Study the drawing (mm; zero at the part's minimum x, y, z) and answer. A direction names the side the tool comes from. Give positions to 0.01 mm unless a question says otherwise; leave off trailing zeros. Order: outer loops, then holes, each group sorted by start corner. A loop starts at its lowest first (then second) coordinate and runs counter-clockwise, first axis right, second up. Notation, with made-up numbers: (-4.75, 29) - (45.25, 29) arc R23 cw to (45.25, 58) - close; hole circle Ø5 at (-19.75, -9). An arc over 180 degrees is marked (long way). Write each question's results on one line, items separated by ' | '. Start each with the question number.
1. Flat-ended cylindrical pins translate along their axes: pin 1 (6.5 mm diameter, centred on x = 10, y = 24, fed in from +Z); pin 2 (12 mm diameter, centred on y = 21, z = 6, fed in from +X); pin 3 (2 mm diameter, centred on y = 6.5, z = 11.5, fed in from -X); pin 4 (6 mm diameter, centred on x = 64, y = 24, fed in from -Z). Find the tip coordinate at first contact, or state that the pin passes through.
2. Section A-A (y = 24) is taken. Give the vertices of the cut face in (x, z), and give its area (3 significant figures).
3. Section D-D (y = 6) is taken. Give the vertices of the cut face in (x, z).
4. Section B-B (z = 20) is taken. Give the vertices of the cut face in (x, y).
5. Section C-C (x = 49) is taken. Give the vertices of the cut face in (y, z), and give its area (3 significant figures).
6. Determine the mould class of the marked faces 4, 5, 6 and 7 for opening direction X: released by +X, released by -X, zero draft, split by the parting line, or undercut.
7. Find the intervals of material crossed by L1, parallel to Y at x = 49, z = 0.9; L2, parallel to X at y = 16.75, z = 16; L3, parallel to Z at x = 28, y = 24.5, in increasing order.
8. Which of the six approach directions +Z, -Z, +X, -X, +Y, -Y give full straight-line access (tool end or side, diameter ignored) to the marked faces 1, 2 and 3?
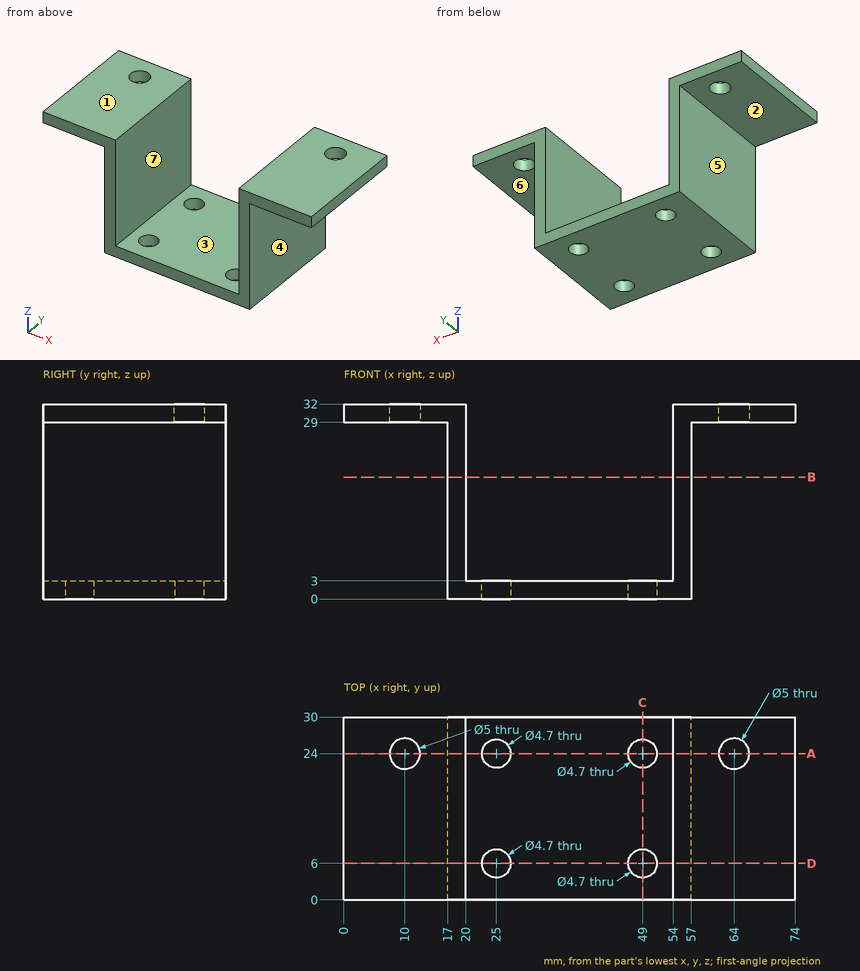
Reported:
1) pin 1: z = 32 | pin 2: x = 57 | pin 3: x = 17 | pin 4: z = 29
2) outline: (0, 29) - (7.5, 29) - (7.5, 32) - (0, 32) - close; (12.5, 29) - (17, 29) - (17, 0) - (22.65, 0) - (22.65, 3) - (20, 3) - (20, 32) - (12.5, 32) - close; (27.35, 0) - (46.65, 0) - (46.65, 3) - (27.35, 3) - close; (51.35, 0) - (57, 0) - (57, 29) - (61.5, 29) - (61.5, 32) - (54, 32) - (54, 3) - (51.35, 3) - close; (66.5, 29) - (74, 29) - (74, 32) - (66.5, 32) - close | area: 338 mm²
3) outline: (0, 29) - (17, 29) - (17, 0) - (22.65, 0) - (22.65, 3) - (20, 3) - (20, 32) - (0, 32) - close; (27.35, 0) - (46.65, 0) - (46.65, 3) - (27.35, 3) - close; (51.35, 0) - (57, 0) - (57, 29) - (74, 29) - (74, 32) - (54, 32) - (54, 3) - (51.35, 3) - close
4) outline: (17, 0) - (20, 0) - (20, 30) - (17, 30) - close; (54, 0) - (57, 0) - (57, 30) - (54, 30) - close
5) outline: (0, 0) - (3.65, 0) - (3.65, 3) - (0, 3) - close; (8.35, 0) - (21.65, 0) - (21.65, 3) - (8.35, 3) - close; (26.35, 0) - (30, 0) - (30, 3) - (26.35, 3) - close | area: 61.8 mm²
6) face 4: released by +X | face 5: released by -X | face 6: zero draft | face 7: undercut
7) L1: 0 to 3.65, 8.35 to 21.65, 26.35 to 30 | L2: 17 to 20, 54 to 57 | L3: 0 to 3
8) face 1: +Z, +X, -X, +Y, -Y | face 2: -Z, -X, +Y, -Y | face 3: +Z, +Y, -Y
